from build123d import *

# Parameters (mm, degrees)
AUFSATZ_LINEAR_AUSTRAGEN1_DEPTH = 5


with BuildPart() as part:
    # Skizze1 → Aufsatz-Linear austragen1 (new body)
    with BuildSketch(Plane.XY):
        Polygon((430.89618142, 326.340211581), (430.89618142, 336.340211581), (425.89618142, 336.340211581), (425.89618142, 346.340211581), (430.89618142, 346.340211581), (430.89618142, 356.340211581), (425.89618142, 356.340211581), (425.89618142, 366.340211581), (430.89618142, 366.340211581), (430.89618142, 376.340211581), (425.89618142, 376.340211581), (425.89618142, 386.340211581), (430.89618142, 386.340211581), (430.89618142, 396.340211581), (425.89618142, 396.340211581), (425.89618142, 406.340211581), (430.89618142, 406.340211581), (430.89618142, 416.340211581), (425.89618142, 416.340211581), (425.89618142, 426.340211581), (430.89618142, 426.340211581), (430.89618142, 436.340211581), (425.89618142, 436.340211581), (425.89618142, 446.340211581), (430.89618142, 446.340211581), (430.89618142, 456.340211581), (425.89618142, 456.340211581), (425.89618142, 466.340211581), (430.89618142, 466.340211581), (430.89618142, 476.340211581), (425.89618142, 476.340211581), (425.89618142, 486.340211581), (430.89618142, 486.340211581), (430.89618142, 496.340211581), (425.89618142, 496.340211581), (425.89618142, 506.340211581), (430.89618142, 506.340211581), (430.89618142, 516.340211581), (425.89618142, 516.340211581), (425.89618142, 526.340211581), (430.89618142, 526.340211581), (430.89618142, 536.340211581), (460.89618142, 566.340211581), (700.89618142, 566.340211581), (730.89618142, 536.340211581), (730.89618142, 526.340211581), (735.89618142, 526.340211581), (735.89618142, 516.340211581), (730.89618142, 516.340211581), (730.89618142, 506.340211581), (735.89618142, 506.340211581), (735.89618142, 496.340211581), (730.89618142, 496.340211581), (730.89618142, 486.340211581), (735.89618142, 486.340211581), (735.89618142, 476.340211581), (730.89618142, 476.340211581), (730.89618142, 466.340211581), (735.89618142, 466.340211581), (735.89618142, 456.340211581), (730.89618142, 456.340211581), (730.89618142, 446.340211581), (735.89618142, 446.340211581), (735.89618142, 436.340211581), (730.89618142, 436.340211581), (730.89618142, 426.340211581), (735.89618142, 426.340211581), (735.89618142, 416.340211581), (730.89618142, 416.340211581), (730.89618142, 406.340211581), (735.89618142, 406.340211581), (735.89618142, 396.340211581), (730.89618142, 396.340211581), (730.89618142, 386.340211581), (735.89618142, 386.340211581), (735.89618142, 376.340211581), (730.89618142, 376.340211581), (730.89618142, 366.340211581), (735.89618142, 366.340211581), (735.89618142, 356.340211581), (730.89618142, 356.340211581), (730.89618142, 346.340211581), (735.89618142, 346.340211581), (735.89618142, 336.340211581), (730.89618142, 336.340211581), (730.89618142, 326.340211581), (735.89618142, 326.340211581), (735.89618142, 316.340211581), (730.89618142, 316.340211581), (430.89618142, 316.340211581), (425.89618142, 316.340211581), (425.89618142, 326.340211581), align=None)
        Polygon((700.89618142, 505.311376979), (670.89618142, 535.311376979), (490.89618142, 535.311376979), (460.89618142, 505.311376979), (460.89618142, 395.311376979), (700.89618142, 395.311376979), align=None, mode=Mode.SUBTRACT)
    extrude(amount=AUFSATZ_LINEAR_AUSTRAGEN1_DEPTH)


solid = part.part
The model under review builds one solid part; all positions refer to its coordinate system, in mm. A direction names the side the tool comes from. Round coordinates to 2 decimals unless told otherwise and drop trailing zeros. Write each loop counter-clockwise with the first axis right and the second up, starting at its lowest first coordinate (ties: lowest second). Pieces come first, ordered by that corner, then holes. Notation, with made-up numbers: (32.25, 84.5) -> (57.25, 84.5) arc R28 cw to (57.25, 123.5) -> close; hole circle Ø9 at (2.25, -24.75). An arc over 180 degrees is marked (long way). Answer as a JSON object with one key per item and string values.
1. We need section B-B on x = 543.5. State the section outline as (y, z) points, and give its area (3 significant figures).
Results found:
{"outline": "(316.34, 0) -> (395.31, 0) -> (395.31, 5) -> (316.34, 5) -> close; (535.31, 0) -> (566.34, 0) -> (566.34, 5) -> (535.31, 5) -> close", "area": "550 mm^2"}
2. Machinability: for faces 1 (the face through (686.11, 520.1, 2.46)), 2 (the face through (583, 388, 0)), which of the approach directions +Z, -Z, +X, -X, +Y, -Y give a long, thin tool a straight path to every point of the face, cutting with its end or side? Answer none if there is none.
Results found:
{"face 1": "+Z, -Z", "face 2": "-Z, +X, -X, +Y, -Y"}
3. We need section A-A on y = 452.5. State the section outline as (x, z) points, and give its area (3 significant figures).
Results found:
{"outline": "(430.9, 0) -> (460.9, 0) -> (460.9, 5) -> (430.9, 5) -> close; (700.9, 0) -> (730.9, 0) -> (730.9, 5) -> (700.9, 5) -> close", "area": "300 mm^2"}
4. The part is to be moulded in two halves that separate along X. For faces 3 (the face through (476.106, 520.521, 2.465)), 4 (the face through (715.686, 551.55, 2.465)), 5 (the face through (583, 388, 5)), say which applies: pulls with the +X half, pulls with the -X half, needs draft (parallel to the pull), parting line crosses it, or undercut.
Results found:
{"face 3": "undercut", "face 4": "pulls with the +X half", "face 5": "needs draft"}
5. Clearance check with flat-ended pins moving along their axes: pin 1 (2.5 mm diameter, centred on x = 734.5, z = 1.5, fed in from +Y); pin 2 (1.5 mm diameter, centred on y = 392.5, z = 4, fed in from -X); pin 3 (10 mm diameter, centred on x = 479, y = 515, fed in from +Z). State where each tip first meets the part, or that it passes through.
Results found:
{"pin 1": "stops at y = 526.34", "pin 2": "stops at x = 430.9", "pin 3": "passes through"}
6. We need section C-C on x = 451.5. State the section outline as (y, z) points.
Results found:
{"outline": "(316.34, 0) -> (556.94, 0) -> (556.94, 5) -> (316.34, 5) -> close"}
7. To check wall thickness, follow line 1 along Y through (x, z) = (511, 3.1); line 2 along X through (y, z) = (405, 4.35); line 3 along X through (y, z) = (494, 4.6). State the ranges of each line that lie inside material, in increasing order.
Results found:
{"line 1": "y = 316.34 to 395.31, 535.31 to 566.34", "line 2": "x = 425.9 to 460.9, 700.9 to 735.9", "line 3": "x = 430.9 to 460.9, 700.9 to 730.9"}
